Could you check a few things on this model? Use its own coordinates, in mm. Give positions to 0.01 mm unless a question says otherwise; leave off trailing zeros. Write each loop counter-clockwise with the first axis right and the second up, starting at its lowest first coordinate (ties: lowest second). Pieces come first, ordered by that corner, then holes. Notation, with made-up numbers: (14.25, 46.5) - (26.25, 46.5) arc R32 ccw to (26.25, 80.5) - close; hole circle Ø3 at (49.5, 73). An arc over 180 degrees is marked (long way). Use one line per item in the form item = value.
```python
from build123d import *

# Parameters (mm, degrees)
F0_W     = 303.70272
F0_H     = 378.451567
F1_DEPTH = 3.41884
F2_R     = 3.96875
F3_R     = 1.35255
F3_W     = 169.31132
F3_H     = 206.951268
F4_DEPTH = 3.41884
F5_R     = 1.8288
F6_DEPTH = 3.41884


with BuildPart() as f1:
    # F0 (on Top) → F1 (new body)
    with BuildSketch(Plane.XY):
        with Locations((-151.85136, -189.225783)):
            Rectangle(F0_W, F0_H)
    extrude(amount=F1_DEPTH)

    # F2
    f2_edges = [f1.edges().sort_by_distance(p)[0] for p in [
        (-303.70272, 0, 1.70942),
        (-303.70272, -378.451567, 1.70942),
        (0, -378.451567, 1.70942),
        (0, 0, 1.70942),
    ]]
    fillet(f2_edges, radius=F2_R)

    # F3 (on face) → F4 (cut, through all)
    with BuildSketch(Plane.XY.offset(3.41884)):
        with Locations((-299.73397, -3.96875)):
            Circle(F3_R)
        with Locations((-3.96875, -3.96875)):
            Circle(F3_R)
        with Locations((-299.73397, -374.482817)):
            Circle(F3_R)
        with Locations((-3.96875, -374.482817)):
            Circle(F3_R)
        with Locations((-286.54629, -34.632519)):
            Circle(F3_R)
        with Locations((-17.15643, -34.632519)):
            Circle(F3_R)
        with Locations((-132.182794, -149.463223)):
            Rectangle(F3_W, F3_H)
    extrude(amount=-F4_DEPTH, mode=Mode.SUBTRACT)

    # F5 (on face) → F6 (cut, through all)
    with BuildSketch(Plane.XY.offset(3.41884)):
        with Locations((-286.54629, -374.482817)):
            Circle(F5_R)
        with Locations((-17.15643, -374.482817)):
            Circle(F5_R)
    extrude(amount=-F6_DEPTH, mode=Mode.SUBTRACT)


solid = f1.part
```
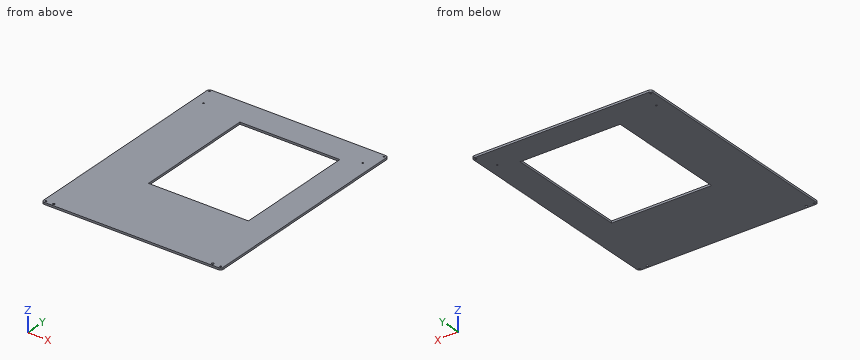
1. If I drill on line 1 (X direction, y = -103.5, z = 0.85); line 2 (Y direction, x = -181.5, z = 3), over which ranges is the centre line in solid material (lowest first)? Write a range as from..to.
Response values:
line_1 = -303.7..-216.84, -47.53..0
line_2 = -378.45..-252.94, -45.99..0
2. Imagine slicing it at C-C, the plane z = 1.85. State how many separate pieces and enclosed holes the cut face has, and give its area (3 significant figures).
Response values:
separate_pieces = 1
enclosed_holes = 9
area = 79,800 mm²
3. Imagine slicing it at A-A, the plane y = -89. List the corners of the cut face in (x, z) for me.
Response values:
outline = (-303.7, 0) - (-216.84, 0) - (-216.84, 3.42) - (-303.7, 3.42) - close; (-47.53, 0) - (0, 0) - (0, 3.42) - (-47.53, 3.42) - close
4. Imagine slicing it at B-B, the plane x = -110.5. List the corners of the cut face in (y, z) for me, and give its area (3 significant figures).
Response values:
outline = (-378.45, 0) - (-252.94, 0) - (-252.94, 3.42) - (-378.45, 3.42) - close; (-45.99, 0) - (0, 0) - (0, 3.42) - (-45.99, 3.42) - close
area = 586 mm²
